```python
from build123d import *

# Parameters (mm, degrees)
SKETCH2_R           = 12.6
BOSS_EXTRUDE1_DEPTH = 5.4
SKETCH3_R           = 1.05
SKETCH3_R_2         = 2.6
CUT_EXTRUDE1_DEPTH  = 413.785561763


with BuildPart() as part:
    # Sketch2 → Boss-Extrude1 (new body)
    with BuildSketch(Plane.XY):
        with BuildLine():
            Line((-65, 20), (65, 20))
            ThreePointArc((65, 20), (29.659714989, 104.34714566), (17.6, 195))
            Line((17.6, 195), (17.6, 390))
            ThreePointArc((17.6, 390), (0, 407.6), (-17.6, 390))
            Line((-17.6, 390), (-17.6, 195))
            ThreePointArc((-17.6, 195), (-29.659714989, 104.34714566), (-65, 20))
        make_face()
        with Locations((0, 390)):
            Circle(SKETCH2_R, mode=Mode.SUBTRACT)
    extrude(amount=-BOSS_EXTRUDE1_DEPTH)

    # Sketch3 → Cut-Extrude1 (cut, through all)
    with BuildSketch(Plane(origin=(0, 0, -5.4), x_dir=(-1, 0, 0), z_dir=(0, 0, -1))):
        with Locations((10.677312396, 400.677312396)):
            Circle(SKETCH3_R)
        with Locations((0, 405.1)):
            Circle(SKETCH3_R)
        with Locations((-10.677312396, 400.677312396)):
            Circle(SKETCH3_R)
        with Locations((-15.1, 390)):
            Circle(SKETCH3_R)
        with Locations((-10.677312396, 379.322687604)):
            Circle(SKETCH3_R)
        with Locations((0, 374.9)):
            Circle(SKETCH3_R)
        with Locations((10.677312396, 379.322687604)):
            Circle(SKETCH3_R)
        with Locations((15.1, 390)):
            Circle(SKETCH3_R)
        with Locations((0, 262.1)):
            Circle(SKETCH3_R_2)
        with Locations((0, 318.7)):
            Circle(SKETCH3_R_2)
        with Locations((-36.174923221, 41.087461611)):
            Circle(SKETCH3_R_2)
        with Locations((36.174923221, 41.087461611)):
            Circle(SKETCH3_R_2)
        with Locations((0, 77.262384832)):
            Circle(SKETCH3_R_2)
        with Locations((0, 117.98239975)):
            Circle(SKETCH3_R_2)
        with Locations((0, 205.5)):
            Circle(SKETCH3_R_2)
    extrude(amount=-CUT_EXTRUDE1_DEPTH, mode=Mode.SUBTRACT)


solid = part.part
```
For this review, take the finished solid that the model builds, in its own axes (mm). Round coordinates to 2 decimals unless told otherwise and drop trailing zeros. Write each loop counter-clockwise with the first axis right and the second up, starting at its lowest first coordinate (ties: lowest second). Pieces come first, ordered by that corner, then holes. Notation, with made-up numbers: (-8, 71.5) - (0, 71.5) arc R27 cw to (0, 108.5) - close; hole circle Ø2 at (54.25, -36). An arc over 180 degrees is marked (long way). Write each question's results on one line, items separated by ' | '.
Item 1: To check wall thickness, follow line 1 along X through (y, z) = (262.1, -1.35); line 2 along X through (y, z) = (235, -3.6); line 3 along Y through (x, z) = (15.1, -2.95). State the ranges of each line that lie inside material, in increasing order. Write a range as from..to.
Calculated:
line 1: x = -17.6..-2.6, 2.6..17.6 | line 2: x = -17.6..17.6 | line 3: y = 20..388.95, 391.05..399.04
Item 2: Take a section at B-B on x = 44.5. State the section outline as (y, z) points.
Calculated:
outline: (20, -5.4) - (61.09, -5.4) - (61.09, 0) - (20, 0) - close
Item 3: Take a section at A-A on z = -1.75. Count the separate pieces of the cut face and the enclosed holes in it, then the cut area to 3 significant figures.
Calculated:
separate pieces: 1 | enclosed holes: 16 | area: 18,200 mm^2
Item 4: Draft analysis for pull direction X (two halves, no side actions). For faces 1 (the face through (-1, 173, 0)), 2 (the face through (0.387, 407.596, -2.662)), 3 (the face through (-1.6, 402.5, -2.7)), state which applies: pulls with the +X half, pulls with the -X half, needs draft (parallel to the pull), parting line crosses it, or undercut.
Calculated:
face 1: needs draft | face 2: parting line crosses it | face 3: undercut
Item 5: For pin 1 (4.5 mm diameter, centred on x = 36.17, y = 41.09, fed in from +Z); pin 2 (1.6 mm diameter, centred on y = 261, z = -2, fed in from -X); pin 3 (2 mm diameter, centred on y = 98, z = -3.5, fed in from +X), all flat-tipped, find the tip position at first contact; note any pin that passes through.
Calculated:
pin 1: passes through | pin 2: stops at x = -17.6 | pin 3: stops at x = 31.74
Item 6: Take a section at C-C on x = -23. State the section outline as (y, z) points.
Calculated:
outline: (20, -5.4) - (134.04, -5.4) - (134.04, 0) - (20, 0) - close
